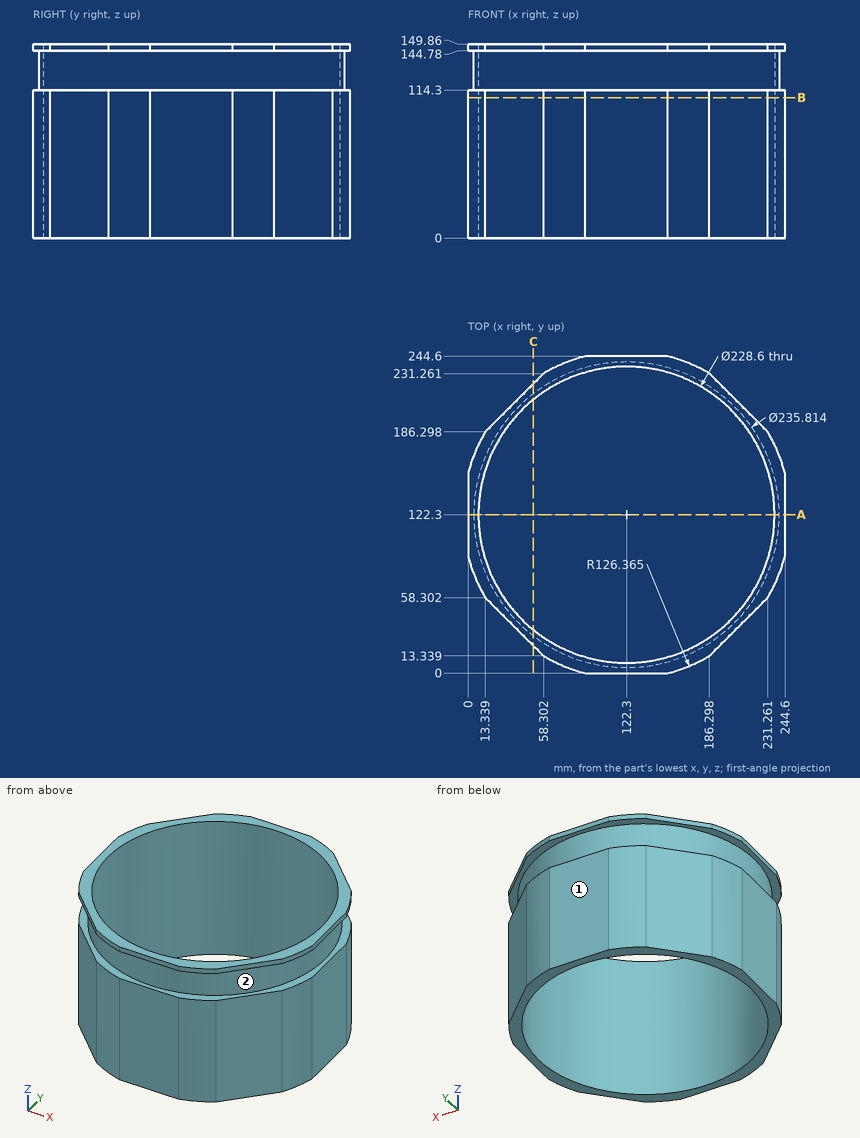
The figure shows three views and two pictorial views of one solid part (mm, origin at its lowest corner). Answer the questions. Coordinates: 2 decimals unless noted, no trailing zeros. Order: outer loops, then holes, each group sorted by start corner. A loop starts at its lowest first (then second) coordinate and runs counter-clockwise, first axis right, second up.
Q1. Consider line 1 (X direction, y = 122, z = 124); line 2 (Z direction, x = 42.5, y = 214). Determine where each line is inside the solid, lowest interval first.
Q2. For a pull along Z with two mould halves and no side action, classify the marked faces 1 and 2 as pulls with the +Z half, pulls with the -Z half, needs draft (parallel to the pull), parting line crosses it, or undercut.
Q3. A cutting plane is placed at A-A, the plane y = 122.3. Write down the section's boundary in (x, z), and give its area (3 significant figures).
Q4. A cutting plane is placed at B-B, the plane z = 108.5. Write down the section's boundary in (x, y) (1 decimal), and give its area (3 significant figures).
Q5. A cutting plane is placed at C-C, the plane x = 50.5. Write down the section's boundary in (y, z) (1 decimal).
Q6. Given P1, Ø10, axis at x = 35.5, z = 79.5, coming from the -Y side; P2, Ø3, axis at x = 105.5, z = 119, coming from the +Y side; P3, Ø6, axis at y = 31.5, z = 59.5, coming from the -X side, each flat-ended and moving along its own axis, determine where each tip first touches the part or whether it passes through.
Answers follow:
1. line 1: x = 4.39 to 8, 236.6 to 240.21
1. line 2: z = 0 to 114.3, 144.78 to 149.86
2. face 1: needs draft
2. face 2: undercut
3. outline: (0, 0) - (8, 0) - (8, 149.86) - (0, 149.86) - (0, 144.78) - (4.39, 144.78) - (4.39, 114.3) - (0, 114.3) - close; (236.6, 0) - (244.6, 0) - (244.6, 114.3) - (240.21, 114.3) - (240.21, 144.78) - (244.6, 144.78) - (244.6, 149.86) - (236.6, 149.86) - close
3. area: 2,130 mm2
4. outline: (0, 90.5) arc R126.4 ccw to (13.3, 58.3) - (58.3, 13.3) arc R126.4 ccw to (90.5, 0) - (154.1, 0) arc R126.4 ccw to (186.3, 13.3) - (231.3, 58.3) arc R126.4 ccw to (244.6, 90.5) - (244.6, 154.1) arc R126.4 ccw to (231.3, 186.3) - (186.3, 231.3) arc R126.4 ccw to (154.1, 244.6) - (90.5, 244.6) arc R126.4 ccw to (58.3, 231.3) - (13.3, 186.3) arc R126.4 ccw to (0, 154.1) - close; hole circle Ø228.6 at (122.3, 122.3)
4. area: 7,740 mm2
5. outline: (21.1, 0) - (33.4, 0) - (33.4, 149.9) - (21.1, 149.9) - (21.1, 144.8) - (28.8, 144.8) - (28.8, 114.3) - (21.1, 114.3) - close; (211.2, 0) - (223.5, 0) - (223.5, 114.3) - (215.8, 114.3) - (215.8, 144.8) - (223.5, 144.8) - (223.5, 149.9) - (211.2, 149.9) - close
6. P1: stops at y = 31.14
6. P2: stops at y = 239.21
6. P3: stops at x = 37.14
